Source: CAD feature listing. Evaluate the final solid. Frame: model axes, mm. A direction names the side the tool comes from. Coordinates: 2 decimals unless noted, no trailing zeros. Order: outer loops, then holes, each group sorted by start corner. A loop starts at its lowest first (then second) coordinate and runs counter-clockwise, first axis right, second up. Notation, with made-up numbers: (14.25, 24) -> (67.25, 24) arc R35 ccw to (67.25, 56) -> close; hole circle Ø5 at (-30, -23). An arc over 180 degrees is marked (long way). Put each result on its own line as item: value.
from build123d import *

# Parameters (mm, degrees)
SKETCH1_W           = 10
SKETCH1_H           = 113
BOSS_EXTRUDE1_DEPTH = 10
BOSS_EXTRUDE2_DEPTH = 5
SKETCH4_W           = 60
SKETCH4_H           = 35
BOSS_EXTRUDE3_DEPTH = 5
BOSS_EXTRUDE4_DEPTH = 5


with BuildPart() as part:
    # Sketch1 → Boss-Extrude1 (new body)
    with BuildSketch(Plane(origin=(0, 0, 0), x_dir=(0, 1, 0), z_dir=(0, 0, 1))):
        Rectangle(SKETCH1_W, SKETCH1_H)
    extrude(amount=BOSS_EXTRUDE1_DEPTH)

    # Sketch3 → Boss-Extrude2 (add)
    with BuildSketch(Plane.YZ.offset(56.5)):
        Polygon((-5, 10), (0, 15), (5, 10), align=None)
    extrude(amount=-BOSS_EXTRUDE2_DEPTH)

    # Sketch4 → Boss-Extrude3 (add)
    with BuildSketch(Plane(origin=(-56.5, 0, 0), x_dir=(0, -1, 0), z_dir=(-1, 0, 0))):
        with Locations((0, 17.5)):
            Rectangle(SKETCH4_W, SKETCH4_H)
    extrude(amount=-BOSS_EXTRUDE3_DEPTH)

    # Sketch5 → Boss-Extrude4 (add)
    with BuildSketch(Plane.YZ.offset(-51.5)):
        Polygon((5, 10), (0, 15), (-5, 10), align=None)
    extrude(amount=BOSS_EXTRUDE4_DEPTH)


solid = part.part
1. Cut plane C-C on y = 14.5. Output: boundary loops of the cut face in (x, z).
Numbers:
outline: (-56.5, 0) -> (-51.5, 0) -> (-51.5, 35) -> (-56.5, 35) -> close
2. Cut plane A-A on z = 12. Output: boundary loops of the cut face in (x, y).
Numbers:
outline: (-56.5, -30) -> (-51.5, -30) -> (-51.5, -3) -> (-46.5, -3) -> (-46.5, 3) -> (-51.5, 3) -> (-51.5, 30) -> (-56.5, 30) -> close; (51.5, -3) -> (56.5, -3) -> (56.5, 3) -> (51.5, 3) -> close
3. First-contact query: pin 1 (10.5 mm diameter, centred on y = -7, z = 16.5, fed in from +X); pin 2 (11 mm diameter, centred on x = -17.5, z = 4, fed in from -Y); pin 3 (3 mm diameter, centred on x = 38, z = 7.5, fed in from +Y). Flat tips, straight axial feed; report the tip coordinate or a pass-through.
Numbers:
pin 1: stops at x = -51.5
pin 2: stops at y = -5
pin 3: stops at y = 5
4. Cut plane B-B on x = 15.5. Output: boundary loops of the cut face in (y, z), plus the area to 3 significant figures.
Numbers:
outline: (-5, 0) -> (5, 0) -> (5, 10) -> (-5, 10) -> close
area: 100 mm2
5. Ray query, line 1 along X through (y, z) = (-7, 26); line 2 along Y through (x, z) = (45, 8). Return the intervals inside material, ascending.
Numbers:
line 1: x = -56.5 to -51.5
line 2: y = -5 to 5
6. Pull-direction query (X, two-part tool) for faces 6 (the flat face through (2, 0, 10)), 7 (the flat face through (-49, 3, 12)), 8 (the flat face through (56.5, 0, 6)); classes: pulls with the +X half, pulls with the -X half, needs draft (parallel to the pull), parting line crosses it, or undercut.
Numbers:
face 6: undercut
face 7: needs draft
face 8: pulls with the +X half
7. Set-up query: faces 1 (the flat face through (3, 5, 5)), 2 (the flat face through (54, 2, 13)), 3 (the flat face through (-49, -2, 13)), 4 (the flat face through (3, -5, 5)), 5 (the flat face through (-46.5, 0, 12)). Return all of +Z, -Z, +X, -X, +Y, -Y with unobstructed straight access to the full face (end or side cutting, diameter ignored); none if empty.
Numbers:
face 1: +Z, -Z, +X, +Y
face 2: +Z, +X, +Y
face 3: +Z, +X, -Y
face 4: +Z, -Z, +X, -Y
face 5: +Z, +Y, -Y
